Input: part model. Units: mm. Frame: model coordinates. A direction names the side the tool comes from. Round coordinates to 2 decimals unless told otherwise and drop trailing zeros. Loops run counter-clockwise (first coordinate to the right, second up) from the corner with the lowest first, then second, coordinate; pieces in that order, holes last. Notation, with made-up numbers: (-20, 18) - (38, 18) arc R28 cw to (38, 42) - close; hole circle Ø7 at (34, -36.5). An arc over 180 degrees is marked (long way). Use CSV: the item, a comma, the result in double quotes. Start each with the question number.
1. Cut plane B-B (z = 10). Return loops of the section in (x, y).
2. Access query for faces 1 (the flat face through (0, -6.5, 11)), 2 (the flat face through (0, 8.5, 10)), 3 (the flat face through (13, 0, 7)), 4 (the flat face through (-2, 0, 2)), 5 (the flat face through (-14, 0, 10)). Directions: +Z, -Z, +X, -X, +Y, -Y. A direction counts if a zero-diameter tool reaches every point of the face in a straight line with its end or side. Return the directions, or none.
3. Pull-direction query (Y, two-part tool) for faces 6 (the flat face through (0, -8.5, 10)), 7 (the flat face through (14, 0, 12)), 8 (the flat face through (9, 0, 1)), 9 (the flat face through (12, 0, 13)); classes: +Y half, -Y half, draft (parallel to the pull), parting line (faces both ways), or undercut.
4. Cut plane D-D (x = -6.5). Return loops of the section in (y, z).
5. Pin query (flat end, axial travel): P1, Ø1.5, axis at x = 12.5, y = -3.5, coming from the -Z side; P2, Ø4, axis at x = -1, y = 2.5, coming from the +Z side; P3, Ø3.5, axis at y = 3, z = 5, coming from the +X side. Return the tip coordinate at first contact, or that it passes through.
6. Cut plane A-A (y = -5.75). Return loops of the section in (x, z), and give its area (3 significant figures).
7. Cut plane C-C (z = 6.25). Return loops of the section in (x, y).
8. Material intervals for probe 1 along Y at (x, z) = (-10.75, 6); probe 2 along X at (y, z) = (1.25, 7.25); probe 3 along Z at (x, y) = (7.25, 6), sorted ascending. Write a range as from..to.
```python
from build123d import *

# Parameters (mm, degrees)
F0_W     = 28
F0_H     = 17
F1_DEPTH = 20
F2_T     = -2
F3_W     = 14
F3_H     = 5
F4_DEPTH = 5
F5_DEPTH = 2


with BuildPart() as f1:
    # F0 (on Top) → F1 (new body)
    with BuildSketch(Plane.XY):
        Rectangle(F0_W, F0_H)
    extrude(amount=F1_DEPTH)

    # F2
    f2_openings = [f1.faces().sort_by_distance(p)[0] for p in [
        (0, 0, 20),
    ]]
    offset(amount=F2_T, openings=f2_openings)

    # F3 (on face) → F4 (cut)
    with BuildSketch(Plane.YZ.offset(14)):
        with Locations((0, 2.5)):
            Rectangle(F3_W, F3_H)
    extrude(amount=-F4_DEPTH, mode=Mode.SUBTRACT)

    # F5 (cut): a face of the model
    f5_faces = [f1.faces().sort_by_distance(p)[0] for p in [
        (12.7580645161, 0, 5),
    ]]
    extrude(f5_faces, amount=-F5_DEPTH, mode=Mode.SUBTRACT)


solid = f1.part
```
Established:
1,outline,"(-14, -8.5) - (14, -8.5) - (14, 8.5) - (-14, 8.5) - close; hole (-12, -6.5) - (12, -6.5) - (12, 6.5) - (-12, 6.5) - close"
2,face 1,"+Z"
2,face 2,"+Z, -Z, +X, -X, +Y"
2,face 3,"-Z, +X"
2,face 4,"+Z, +X"
2,face 5,"+Z, -Z, -X, +Y, -Y"
3,face 6,"-Y half"
3,face 7,"draft"
3,face 8,"undercut"
3,face 9,"undercut"
4,outline,"(-8.5, 0) - (8.5, 0) - (8.5, 20) - (6.5, 20) - (6.5, 2) - (-6.5, 2) - (-6.5, 20) - (-8.5, 20) - close"
5,P1,"stops at z = 7"
5,P2,"stops at z = 2"
5,P3,"stops at x = -12"
6,outline,"(-14, 0) - (9, 0) - (9, 2) - (-12, 2) - (-12, 20) - (-14, 20) - close; (12, 7) - (14, 7) - (14, 20) - (12, 20) - close"
6,area,"108 mm2"
7,outline,"(-14, -8.5) - (14, -8.5) - (14, -7) - (9, -7) - (9, -6.5) - (-12, -6.5) - (-12, 6.5) - (9, 6.5) - (9, 7) - (14, 7) - (14, 8.5) - (-14, 8.5) - close"
8,probe 1,"y = -8.5..-6.5, 6.5..8.5"
8,probe 2,"x = -14..-12, 12..14"
8,probe 3,"z = 0..2"
